Build history of the part. All positions in model axes, mm. Give positions to 0.01 mm unless a question says otherwise; leave off trailing zeros. Loops run counter-clockwise (first coordinate to the right, second up) from the corner with the lowest first, then second, coordinate; pieces in that order, holes last. Notation, with made-up numbers: (56, 6.25) - (109, 6.25) arc R33 cw to (109, 42.25) - close; hole circle Ø8 at (12.5, 84). An arc over 180 degrees is marked (long way). Return JSON: item names as keys, results as strings. Group by question number.
1) Mould opens along X. For faces 1 (the face through (-17, 13.5, 4.9)), 2 (the face through (-1, 30, 5)), 3 (the face through (70, 0, 5)) say: released by +X, released by -X, zero draft, split by the parting line, or undercut.
2) Slice it at B-B (x = -65). List the corners of the cut face in (y, z), and give its area (3 significant figures).
3) Slice it at D-D (z = 2.5). Count the separate pieces of the cut face and the enclosed holes in it, and give its area (3 significant figures).
4) Slice it at C-C (y = 0). List the corners of the cut face in (x, z).
5) Slice it at A-A (x = 50). List the corners of the cut face in (y, z), and give its area (3 significant figures).
6) Drill centre lines: probe 1 along Y at (x, z) = (15, 5.75); probe 2 along Y at (x, z) = (-65, 6.75); probe 3 along Y at (x, z) = (51.5, 8.75). Where is each one in solid material? Low to high. Write a range as from..to.
```python
from build123d import *

# Parameters (mm, degrees)
SKETCH_1_W      = 140
SKETCH_1_H      = 60
SKETCH_1_R      = 2
SKETCH_1_R_2    = 2.5
EXTRUDE_1_DEPTH = 10


with BuildPart() as part:
    # Эскиз1 → Бобышка-Вытянуть1 (new body)
    with BuildSketch(Plane.XY):
        Rectangle(SKETCH_1_W, SKETCH_1_H)
        with Locations((-65, 0)):
            Circle(SKETCH_1_R, mode=Mode.SUBTRACT)
        with Locations((-65, 20)):
            Circle(SKETCH_1_R, mode=Mode.SUBTRACT)
        with Locations((-65, -20)):
            Circle(SKETCH_1_R, mode=Mode.SUBTRACT)
        with Locations(Location((65, -20, 0), (0, 0, 180))):
            Circle(SKETCH_1_R, mode=Mode.SUBTRACT)
        with Locations(Location((65, 20, 0), (0, 0, 180))):
            Circle(SKETCH_1_R, mode=Mode.SUBTRACT)
        with Locations(Location((65, 0, 0), (0, 0, 180))):
            Circle(SKETCH_1_R, mode=Mode.SUBTRACT)
        with Locations((-50, 15)):
            Circle(SKETCH_1_R_2, mode=Mode.SUBTRACT)
        with Locations((-50, -15)):
            Circle(SKETCH_1_R_2, mode=Mode.SUBTRACT)
        with Locations((-15, 15)):
            Circle(SKETCH_1_R_2, mode=Mode.SUBTRACT)
        with Locations((-15, -15)):
            Circle(SKETCH_1_R_2, mode=Mode.SUBTRACT)
        with Locations(Location((15, -15, 0), (0, 0, 180))):
            Circle(SKETCH_1_R_2, mode=Mode.SUBTRACT)
        with Locations(Location((15, 15, 0), (0, 0, 180))):
            Circle(SKETCH_1_R_2, mode=Mode.SUBTRACT)
        with Locations(Location((50, -15, 0), (0, 0, 180))):
            Circle(SKETCH_1_R_2, mode=Mode.SUBTRACT)
        with Locations(Location((50, 15, 0), (0, 0, 180))):
            Circle(SKETCH_1_R_2, mode=Mode.SUBTRACT)
    extrude(amount=EXTRUDE_1_DEPTH)


solid = part.part
```
Results:
{
 "1": {"face 1": "undercut", "face 2": "zero draft", "face 3": "released by +X"},
 "2": {"outline": "(-30, 0) - (-22, 0) - (-22, 10) - (-30, 10) - close; (-18, 0) - (-2, 0) - (-2, 10) - (-18, 10) - close; (2, 0) - (18, 0) - (18, 10) - (2, 10) - close; (22, 0) - (30, 0) - (30, 10) - (22, 10) - close", "area": "480 mm2"},
 "3": {"separate pieces": "1", "enclosed holes": "14", "area": "8,170 mm2"},
 "4": {"outline": "(-70, 0) - (-67, 0) - (-67, 10) - (-70, 10) - close; (-63, 0) - (63, 0) - (63, 10) - (-63, 10) - close; (67, 0) - (70, 0) - (70, 10) - (67, 10) - close"},
 "5": {"outline": "(-30, 0) - (-17.5, 0) - (-17.5, 10) - (-30, 10) - close; (-12.5, 0) - (12.5, 0) - (12.5, 10) - (-12.5, 10) - close; (17.5, 0) - (30, 0) - (30, 10) - (17.5, 10) - close", "area": "500 mm2"},
 "6": {"probe 1": "-30..-17.5, -12.5..12.5, 17.5..30", "probe 2": "-30..-22, -18..-2, 2..18, 22..30", "probe 3": "-30..-17, -13..13, 17..30"}
}
